```python
from build123d import *

# Parameters (mm, degrees)
SKETCH1_R               = 1.397
BOSS_EXTRUDE1_DEPTH     = 18.796
BOSS_EXTRUDE2_DEPTH     = 5.08
SKETCH3_W               = 7.62
SKETCH3_H               = 8.763
BOSS_EXTRUDE3_DEPTH     = 23.876
FILLET1_R               = 0.508
BOSS_EXTRUDE5_DEPTH     = 47.752
FILLET3_R               = 0.508
CUT_EXTRUDE2_DEPTH      = 43.370253148
CUT_EXTRUDE2_DEPTH_BACK = 43.370253148
SKETCH9_W               = 7.62
SKETCH9_H               = 12.7
FILLET4_R               = 0.762
CUT_EXTRUDE3_DEPTH      = 59.837744517
CUT_EXTRUDE3_DEPTH_BACK = 15.494
SKETCH10_R              = 2.921
CUT_EXTRUDE4_DEPTH      = 48.140271953
CUT_EXTRUDE4_DEPTH_BACK = 48.140271953
SKETCH11_R              = 1.7145
CUT_EXTRUDE5_DEPTH      = 59.837744517
CUT_EXTRUDE5_DEPTH_BACK = 15.494
SKETCH12_R              = 3.3655


with BuildPart() as part:
    # Sketch1 → Boss-Extrude1 (new body)
    with BuildSketch(Plane(origin=(0, 0, 0), x_dir=(1, 0, 0), z_dir=(0, 1, 0))):
        with Locations(Location((0, 0, 0), (0, 0, 270))):
            Circle(SKETCH1_R)
    extrude(amount=BOSS_EXTRUDE1_DEPTH)

    # Sketch2 → Boss-Extrude2 (add)
    with BuildSketch(Plane(origin=(0, 18.796, 0), x_dir=(1, 0, 0), z_dir=(0, 1, 0))):
        with BuildLine():
            Line((-3.81, -6.35), (3.81, -6.35))
            Line((3.81, -6.35), (3.81, 0))
            ThreePointArc((3.81, 0), (0, 3.81), (-3.81, 0))
            Line((-3.81, 0), (-3.81, -6.35))
        make_face()
    extrude(amount=BOSS_EXTRUDE2_DEPTH)

    # Sketch3 → Boss-Extrude3 (add)
    with BuildSketch(Plane(origin=(0, 23.876, 0), x_dir=(1, 0, 0), z_dir=(0, 1, 0))):
        with Locations((0, -10.7315)):
            Rectangle(SKETCH3_W, SKETCH3_H)
    extrude(amount=-BOSS_EXTRUDE3_DEPTH)

    # Mirror1: part across plane


with BuildPart() as part_1:
    add(part.part)
    add(part.part.mirror(Plane.ZX))

    # Fillet1
    fillet1_edges = [part_1.edges().sort_by_distance(p)[0] for p in [
        (-3.81, -23.876, 7.5565),
        (3.81, -23.876, 7.5565),
        (0, -23.876, -3.81),
        (-3.81, 23.876, 7.5565),
        (3.81, 23.876, 7.5565),
        (0, 23.876, -3.81),
    ]]
    fillet(fillet1_edges, radius=FILLET1_R)

    # Sketch8 → Boss-Extrude5 (add)
    with BuildSketch(Plane(origin=(0, 23.876, 0), x_dir=(1, 0, 0), z_dir=(0, 1, 0))):
        with BuildLine():
            Line((-3.81, -15.113), (3.81, -15.113))
            Line((3.81, -15.113), (3.81, -30.353))
            ThreePointArc((3.81, -30.353), (0, -34.163), (-3.81, -30.353))
            Line((-3.81, -30.353), (-3.81, -15.113))
        make_face()
    extrude(amount=-BOSS_EXTRUDE5_DEPTH)

    # Fillet3
    fillet3_edges = [part_1.edges().sort_by_distance(p)[0] for p in [
        (-3.81, 23.876, 22.733),
        (0, 23.876, 34.163),
        (3.81, 23.876, 22.733),
        (0, -23.876, 34.163),
        (3.81, -23.876, 22.733),
        (-3.81, -23.876, 22.733),
    ]]
    fillet(fillet3_edges, radius=FILLET3_R)

    # Sketch9 → Cut-Extrude2 (cut, two sides: drawn at the far end of the back side and taken through both)
    with BuildSketch(Plane.ZY.offset(3.81).offset(-CUT_EXTRUDE2_DEPTH_BACK)):
        with Locations((30.353, 0)):
            Rectangle(SKETCH9_W, SKETCH9_H)
    extrude(amount=CUT_EXTRUDE2_DEPTH + CUT_EXTRUDE2_DEPTH_BACK, mode=Mode.SUBTRACT)

    # Fillet4
    fillet4_edges = [part_1.edges().sort_by_distance(p)[0] for p in [
        (0, 6.35, 34.163),
        (0, -6.35, 34.163),
        (0, -6.35, 26.543),
        (-3.81, 0, 26.543),
        (3.81, 0, 26.543),
        (-3.81, -6.35, 28.448),
        (3.81, -6.35, 28.448),
        (0, 6.35, 26.543),
        (-3.81, 6.35, 28.448),
        (3.81, 6.35, 28.448),
    ]]
    fillet(fillet4_edges, radius=FILLET4_R)

    # Sketch10 → Cut-Extrude3 (cut, two sides: drawn at the far end of the back side and taken through both)
    with BuildSketch(Plane(origin=(0, 23.876, 0), x_dir=(1, 0, 0), z_dir=(0, 1, 0)).offset(-CUT_EXTRUDE3_DEPTH_BACK)):
        with Locations(Location((0, -30.353, 0), (0, 0, 90))):
            Circle(SKETCH10_R)
    extrude(amount=CUT_EXTRUDE3_DEPTH + CUT_EXTRUDE3_DEPTH_BACK, mode=Mode.SUBTRACT)

    # Sketch11 → Cut-Extrude4 (cut, two sides: drawn at the far end of the back side and taken through both)
    with BuildSketch(Plane(origin=(0, 8.382, 0), x_dir=(1, 0, 0), z_dir=(0, 1, 0)).offset(-CUT_EXTRUDE4_DEPTH_BACK)):
        with Locations(Location((0, -30.353, 0), (0, 0, 270))):
            Circle(SKETCH11_R)
    extrude(amount=CUT_EXTRUDE4_DEPTH + CUT_EXTRUDE4_DEPTH_BACK, mode=Mode.SUBTRACT)

    # Sketch12 → Cut-Extrude5 (cut, two sides: drawn at the far end of the back side and taken through both)
    with BuildSketch(Plane.XZ.offset(23.876).offset(-CUT_EXTRUDE5_DEPTH_BACK)):
        with Locations(Location((0, 30.353, 0), (0, 0, 180))):
            Circle(SKETCH12_R)
    extrude(amount=CUT_EXTRUDE5_DEPTH + CUT_EXTRUDE5_DEPTH_BACK, mode=Mode.SUBTRACT)


solid = part_1.part
```
Can you work these out from the model? Positions are in its coordinate system, mm. A direction names the side the tool comes from. Round coordinates to 2 decimals unless told otherwise and drop trailing zeros. Loops run counter-clockwise (first coordinate to the right, second up) from the corner with the lowest first, then second, coordinate; pieces in that order, holes last. Notation, with made-up numbers: M 80.5,75.5 L 99.5,75.5 A15 cw 99.5,81.5 Z; hole C 1,-21 d11. An arc over 180 degrees is marked long. Answer as a JSON object with one key per item and string values. Group by question number.
Q1. Imagine slicing it at D-D, the plane x = 0. Count the separate pieces of the cut face and the enclosed holes in it, then the cut area to 3 significant figures.
Q2. On a 3-axis mill with a long thin cutter (end or side, diameter ignored), from which of +Z, -Z, +X, -X, +Y, -Y can I reach the whole of each face in a straight line? I mean faces 4 (the flat face through (-1.3, -6.35, 29)), 5 (the flat face through (2, 8.382, 30)), 6 (the flat face through (0, 18.796, 2)), 7 (the flat face through (0, 0, 6.35)). Say none if no direction works.
Q3. Imagine slicing it at B-B, the plane z = 4. Please give me the cut outline in (x, y), then the cut area to 3 significant figures.
Q4. Imagine slicing it at C-C, the plane y = -0.5. Please give me the cut outline in (x, z), then the cut area to 3 significant figures.
Q5. Will these pins go through, and if not, where does the flat tip stop? pin 1 (0.6 mm diameter, centred on x = 3.5, y = -23.5, fed in from -Z); pin 2 (1.8 mm diameter, centred on x = 1, y = -0.5, fed in from +Z); pin 3 (2 mm diameter, centred on x = 0, z = 30.353, fed in from -Y); pin 4 (4 mm diameter, centred on y = 2, z = 2.5, fed in from -X).
Q6. We'd pull the mould along X, two halves only. Please class faces 1 (the flat face through (0, -23.876, 13)), 2 (the cylindrical face through (0.73, -16.02, 33.64)), 3 (the cylindrical face through (0.084, 15.354, 34.162)): +X half, -X half, draft (parallel to the pull), parting line (faces both ways), or undercut.
Q7. Imagine slicing it at A-A, the plane y = -9.5. Please give me the cut outline in (x, z), then the cut area to 3 significant figures.
Q8. Please list where these lines run through material, in increasing order: L1, parallel to Y at x = 2.75, z = 3; L2, parallel to Y at x = 1.5, z = 31.5; L3, parallel to Z at x = 0.75, y = -16.5.
Findings:
{
 "1": {"separate pieces": "3", "enclosed holes": "1", "area": "1,230 mm2"},
 "2": {"face 4": "+Z, +X, -X", "face 5": "+Y", "face 6": "none", "face 7": "+X, -X"},
 "3": {"outline": "M -3.81,-23.37 A0.51 ccw -3.3,-23.88 L 3.3,-23.88 A0.51 ccw 3.81,-23.37 L 3.81,-18.8 L -3.81,-18.8 Z; M -3.81,18.8 L 3.81,18.8 L 3.81,23.37 A0.51 ccw 3.3,23.88 L -3.3,23.88 A0.51 ccw -3.81,23.37 Z", "area": "77.2 mm2"},
 "4": {"outline": "M -3.81,6.35 L 3.81,6.35 L 3.81,25.78 A0.76 ccw 3.05,26.54 L -3.05,26.54 A0.76 ccw -3.81,25.78 Z; C 0,0 d2.79", "area": "160 mm2"},
 "5": {"pin 1": "stops at z = -2.05", "pin 2": "stops at z = 26.54", "pin 3": "passes through", "pin 4": "stops at x = -1.3"},
 "6": {"face 1": "draft", "face 2": "undercut", "face 3": "parting line"},
 "7": {"outline": "M -3.81,6.35 L 3.81,6.35 L 3.81,30.35 A3.81 ccw -3.81,30.35 Z; C 0,0 d2.79; hole C 0,30.35 d6.73", "area": "176 mm2"},
 "8": {"L1": "y = -23.88 to -18.8, 18.8 to 23.88", "L2": "y = -8.38 to -6.35, 6.35 to 8.38", "L3": "z = -1.18 to 1.18, 6.35 to 27.07, 33.63 to 34.09"}
}
